Here's how the part is built. I have some questions about the finished solid (model axes, mm). Face numbers are marked on the shaded views. A direction names the side the tool comes from. Round coordinates to 2 decimals unless told otherwise and drop trailing zeros. Write each loop counter-clockwise with the first axis right and the second up, starting at its lowest first coordinate (ties: lowest second). Pieces come first, ordered by that corner, then holes. Notation, with made-up numbers: (-29, -22.75) - (-15, -22.75) arc R23 cw to (-15, -8.75) - close; hole circle Ø2 at (-13.5, 81.25). An arc over 180 degrees is marked (long way). One line per question, with ' | ' between items. Start each with the question number.
(1) If I drill on L1, parallel to X at y = 20.45, z = 1.5; L2, parallel to X at y = 4.5, z = 1.1; L3, parallel to Y at x = -1, z = 1.45, over which ranges is the centre line in solid material (lowest first)?
(2) Will these pins go through, and if not, where does the flat tip stop? pin 1 (1.6 mm diameter, centred on y = 27.5, z = 2, fed in from +X); pin 2 (1.6 mm diameter, centred on x = 5, z = 1.5, fed in from +Y); pin 3 (0.9 mm diameter, centred on x = -15, z = 1.5, fed in from +Y); pin 4 (0.9 mm diameter, centred on x = 10, y = 0, fed in from -Z).
(3) Imagine slicing it at B-B (y = 22). Write out the boundary of the cut face in (x, z).
(4) Thinking about a two-plate mould opening in X: for the marked faces 6 and 7, which applies, pulls with the +X half, pulls with the -X half, needs draft (parallel to the pull), parting line crosses it, or undercut?
(5) Imagine slicing it at A-A (x = 6.5). Write out the boundary of the cut face in (y, z).
(6) Imagine slicing it at C-C (x = -1). Write out the boundary of the cut face in (y, z).
(7) For the marked faces 1, 2, 3, 4 and 5, which set-ups out of +Z, -Z, +X, -X, +Y, -Y let a thin tool reach every point of the face, with its end or its side?
(8) Imagine slicing it at D-D (y = 10.5). Write out the boundary of the cut face in (x, z), plus the area to 3 significant figures.
from build123d import *

# Parameters (mm, degrees)
SKETCH1_W           = 4
SKETCH1_H           = 2
BOSS_EXTRUDE1_DEPTH = 3
SKETCH2_R           = 1
CUT_EXTRUDE1_DEPTH  = 8
FILLET1_R           = 1
FILLET2_R           = 0.5


with BuildPart() as part:
    # Sketch1 → Boss-Extrude1 (new body)
    with BuildSketch(Plane.XY):
        with BuildLine():
            ThreePointArc((12, 13), (13.757359313, 8.757359313), (18, 7))
            Line((18, 7), (18, 0))
            Line((18, 0), (13.5, 0))
            ThreePointArc((13.5, 0), (12.646446609, 0.353553391), (13, -0.5))
            Line((13, -0.5), (13, -3))
            Line((13, -3), (10, -3))
            Line((10, -3), (10, -0.5))
            ThreePointArc((10, -0.5), (10.353553391, 0.353553391), (9.5, 0))
            Line((9.5, 0), (0, 0))
            Line((0, 0), (0, 9))
            Line((0, 9), (2.309401077, 9))
            Line((2.309401077, 9), (4.618802154, 13))
            Line((4.618802154, 13), (12, 13))
        make_face()
        with Locations((5, 4)):
            Rectangle(SKETCH1_W, SKETCH1_H, mode=Mode.SUBTRACT)
    extrude(amount=BOSS_EXTRUDE1_DEPTH)

    # Sketch2 → Cut-Extrude1 (cut)
    with BuildSketch(Plane.XZ):
        with Locations(Location((5, 1.5, 0), (0, 0, 270))):
            Circle(SKETCH2_R)
    extrude(amount=-CUT_EXTRUDE1_DEPTH, mode=Mode.SUBTRACT)

    # Fillet1
    fillet1_edges = [part.edges().sort_by_distance(p)[0] for p in [
        (18, 7, 1.5),
        (18, 0, 1.5),
    ]]
    fillet(fillet1_edges, radius=FILLET1_R)

    # Fillet2
    fillet2_edges = [part.edges().sort_by_distance(p)[0] for p in [
        (11.5, -3, 0),
        (13, -3, 1.5),
        (10, -3, 1.5),
        (11.5, -3, 3),
    ]]
    fillet(fillet2_edges, radius=FILLET2_R)

    # Mirror1: part across plane


with BuildPart() as part_1:
    add(part.part)
    add(part.part.mirror(Plane(origin=(0, 0, 3), x_dir=(0, 0, 1), z_dir=(-1, 0, 0))))

    # Mirror2: part across plane


with BuildPart() as part_2:
    add(part_1.part)
    add(part_1.part.mirror(Plane(origin=(0, 13, 3), x_dir=(0, 0, 1), z_dir=(0, 1, 0))))


solid = part_2.part
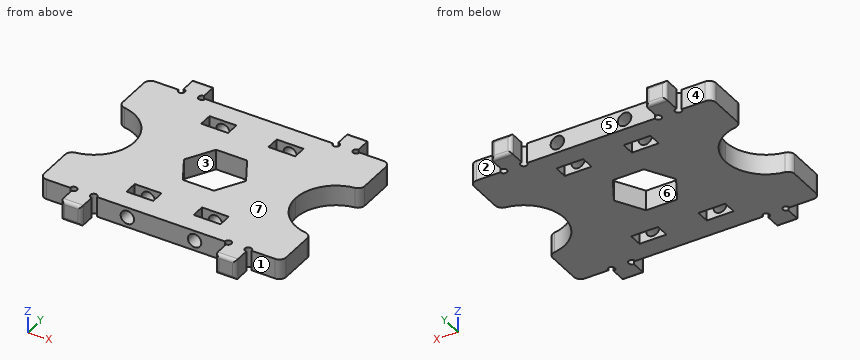
Check sheet entries:
1) L1: -18 to -6, -4 to 4, 6 to 18 | L2: -18 to -7, -3 to 3, 7 to 18 | L3: 0 to 9, 17 to 26
2) pin 1: x = 13 | pin 2: y = 18 | pin 3: y = 26 | pin 4: through
3) outline: (-18, 0) - (-7, 0) - (-7, 3) - (-18, 3) - close; (-3, 0) - (3, 0) - (3, 3) - (-3, 3) - close; (7, 0) - (18, 0) - (18, 3) - (7, 3) - close
4) face 6: undercut | face 7: needs draft
5) outline: (0, 0) - (3, 0) - (3, 3) - (0, 3) - close; (5, 0) - (21, 0) - (21, 3) - (5, 3) - close; (23, 0) - (26, 0) - (26, 3) - (23, 3) - close
6) outline: (0, 0) - (9, 0) - (9, 3) - (0, 3) - close; (17, 0) - (26, 0) - (26, 3) - (17, 3) - close
7) face 1: +Z, -Z, +X, -Y | face 2: +Z, -Z, +X, +Y | face 3: +Z, -Z | face 4: +Z, -Z, -X, +Y | face 5: +Z, -Z, +Y
8) outline: (-12.55, 0) - (-3.18, 0) - (-3.18, 3) - (-12.55, 3) - close; (3.18, 0) - (12.55, 0) - (12.55, 3) - (3.18, 3) - close | area: 56.2 mm^2
